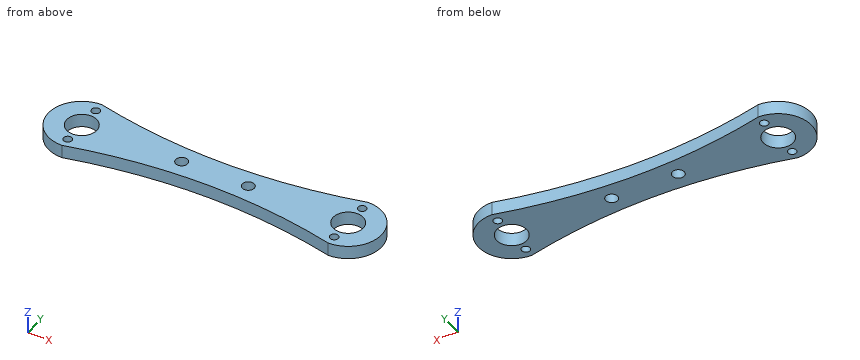
```python
from build123d import *

# Parameters (mm, degrees)
ESQUISSE1_R             = 1.25
ESQUISSE1_R_2           = 4.5
BOSS_EXTRU_1_DEPTH      = 4
ESQUISSE2_R             = 1.8
ENL_V_MAT_EXTRU_1_DEPTH = 10


with BuildPart() as part:
    # Esquisse1 → Boss.-Extru.1 (new body)
    with BuildSketch(Plane.XY):
        with BuildLine():
            ThreePointArc((0, 10.00000024), (-10.00000024, 0), (0, -10.00000024))
            add(Edge.make_bspline(
                [(0, -10.00000024), (40, 0), (80, -10.00000024)],
                knots=[0, 0, 0, 1, 1, 1], degree=2))
            ThreePointArc((80, -10.00000024), (90.00000024, 0), (80, 10.00000024))
            add(Edge.make_bspline(
                [(0, 10.00000024), (40, 0), (80, 10.00000024)],
                knots=[0, 0, 0, 1, 1, 1], degree=2))
        make_face()
        with Locations((80, -7)):
            Circle(ESQUISSE1_R, mode=Mode.SUBTRACT)
        with Locations((80, 7)):
            Circle(ESQUISSE1_R, mode=Mode.SUBTRACT)
        with Locations((0, -7)):
            Circle(ESQUISSE1_R, mode=Mode.SUBTRACT)
        with Locations((0, 7)):
            Circle(ESQUISSE1_R, mode=Mode.SUBTRACT)
        with Locations((80, 0)):
            Circle(ESQUISSE1_R_2, mode=Mode.SUBTRACT)
        Circle(ESQUISSE1_R_2, mode=Mode.SUBTRACT)
    extrude(amount=BOSS_EXTRU_1_DEPTH)

    # Esquisse2 → Enlèv. mat.-Extru.1 (cut)
    with BuildSketch(Plane(origin=(0, 0, 0), x_dir=(-1, 0, 0), z_dir=(0, 0, -1))):
        with Locations((-50, 0)):
            Circle(ESQUISSE2_R)
        with Locations((-30, 0)):
            Circle(ESQUISSE2_R)
    extrude(amount=-ENL_V_MAT_EXTRU_1_DEPTH, mode=Mode.SUBTRACT)


solid = part.part
```
Build history of the part. All positions in model axes, mm. Round coordinates to 2 decimals unless told otherwise and drop trailing zeros. Answer in a Markdown table with one row per item.
1) Band-saw the part on A-A on z = 0.85. Give the number of separate pieces and of enclosed holes in the cut face, and give its area (3 significant figures).
Values:
| item | result |
|---|---|
| separate pieces | 1 |
| enclosed holes | 8 |
| area | 1,210 mm2 |
2) Pin check, flat tips, straight feed: P1, Ø1.5, axis at x = 72.5, z = 2.5, coming from the +Y side; P2, Ø2, axis at x = 19, z = 2.5, coming from the +Y side; P3, Ø1, axis at y = -3, z = 3, coming from the -X side. Stop position of each tip, or through.
Values:
| item | result |
|---|---|
| P1 | y = 8.45 |
| P2 | y = 6.51 |
| P3 | x = -9.68 |
3) Wall check: L1, parallel to Y at x = 80, z = 1.65; L2, parallel to X at y = -3.75, z = 2.95; L3, parallel to Y at x = 80.5, z = 1.95. Give the ranges that are in metal, low to high.
Values:
| item | result |
|---|---|
| L1 | -10 to -8.25, -5.75 to -4.5, 4.5 to 5.75, 8.25 to 10 |
| L2 | -9.27 to -2.49, 2.49 to 77.51, 82.49 to 89.27 |
| L3 | -9.99 to -8.15, -5.85 to -4.47, 4.47 to 5.85, 8.15 to 9.99 |
